Model file for the job. Use its own axes, mm. Give positions to 0.01 mm unless a question says otherwise; leave off trailing zeros. Write each loop counter-clockwise with the first axis right and the second up, starting at its lowest first coordinate (ties: lowest second). Pieces come first, ordered by that corner, then holes. Notation, with made-up numbers: (-21, -31) - (20, -31) arc R28 cw to (20, 5) - close; hole circle Ø5 at (-2.5, -19.75). An arc over 180 degrees is marked (long way). Use a Markdown table: item, result. Add a question column.
```python
from build123d import *

# Parameters (mm, degrees)
SKETCH1_W                   = 174.021305966
SKETCH1_H                   = 271.365530146
BOSS_EXTRUDE1_DEPTH         = 12.7
F_1_4_0_25_DIAMETER_HOLE1_D = 6.35
HOLE1_D                     = 3.175
HOLE1_DEPTH                 = 31.75
HOLE1_CSINK_D               = 10.16
HOLE1_CSINK_ANGLE           = 82
HOLE1_TIP                   = 0.953866233


with BuildPart() as part:
    # Sketch1 → Boss-Extrude1 (new body)
    with BuildSketch(Plane.XY):
        with Locations((212.253144626, 135.682765073)):
            Rectangle(SKETCH1_W, SKETCH1_H)
    extrude(amount=BOSS_EXTRUDE1_DEPTH)

    # 1/4 (0.25) Diameter Hole1 (through all)
    with Locations(Plane(origin=(0, 0, 0), x_dir=(-1, 0, 0), z_dir=(0, 0, -1))):
        with Locations((-277.426568305, 245.965530146), (-211.653264176, 161.082765073), (-150.642491643, 245.965530146), (-211.653264176, 110.282765073), (-277.426568305, 25.4), (-150.642491643, 25.4)):
            Hole(F_1_4_0_25_DIAMETER_HOLE1_D / 2)

    # Hole1
    with Locations(Plane(origin=(-504.900458932, 135.816741379, 12.7), x_dir=(0, -1, 0), z_dir=(0, 0, 1))):
        with Locations((-129.257383629, 766.263727577), (129.466741379, 668.242950575), (129.466741379, 766.064256541), (-129.408220012, 668.442537903)):
            CounterSinkHole(HOLE1_D / 2, HOLE1_CSINK_D / 2, depth=HOLE1_DEPTH, counter_sink_angle=HOLE1_CSINK_ANGLE)
            with Locations((0, 0, -(HOLE1_DEPTH + HOLE1_TIP / 2))):  # 118° drill point
                Cone(0, HOLE1_D / 2, HOLE1_TIP, mode=Mode.SUBTRACT)


solid = part.part
```
(1) Probe probe 1 along Y at (x, z) = (152, 9.5). List the from-to ranges inside material, lowest first. Write a range as [from, to].
(2) Two-plate mould, pull along Y, no slides. Class faces 1 (the cylindrical face through (214.6, 109.1, 6.4)), 2 (the flat face through (211, 138, 12.7)), 3 (the flat face through (211, 0, 6)): +Y half, -Y half, draft (parallel to the pull), parting line (faces both ways), or undercut.
(3) Flat gauge pins, fed straight in: pin 1 (5 mm diameter, centred on x = 163.54, y = 265.22, fed in from -Z); pin 2 (5 mm diameter, centred on x = 261.16, y = 6.35, fed in from +Z); pin 3 (3.5 mm diameter, centred on x = 261.36, y = 265.07, fed in from +Z). Where does each tip first touch, or does it go through?
(4) Band-saw the part on A-A (y = 25.4). Write the cut outline in (x, z), then the cut area to 3 significant figures.
Model answer:
| question | item | result |
|---|---|---|
| 1 | probe 1 | y = [0, 22.53], [28.27, 243.1], [248.84, 271.37] |
| 2 | face 1 | undercut |
| 2 | face 2 | draft |
| 2 | face 3 | -Y half |
| 3 | pin 1 | stops at z = 0 |
| 3 | pin 2 | stops at z = 9.74 |
| 3 | pin 3 | stops at z = 8.88 |
| 4 | outline | (125.24, 0) - (147.47, 0) - (147.47, 12.7) - (125.24, 12.7) - close; (153.82, 0) - (274.25, 0) - (274.25, 12.7) - (153.82, 12.7) - close; (280.6, 0) - (299.26, 0) - (299.26, 12.7) - (280.6, 12.7) - close |
| 4 | area | 2,050 mm^2 |
